```python
from build123d import *

# Parameters (mm, degrees)
SKETCH_1_W      = 20
SKETCH_1_H      = 6
SKETCH_1_W_2    = 6
SKETCH_1_H_2    = 20
EXTRUDE_1_DEPTH = 6


with BuildPart() as part:
    # Эскиз1 → Бобышка-Вытянуть1 (new body)
    with BuildSketch(Plane.XY):
        Polygon((0, 60), (0, 66), (12, 66), (12, 60), (62, 60), (62, 66), (112, 66), (112, 60), (200, 60), (200, 66), (250, 66), (250, 60), (338, 60), (338, 66), (388, 66), (388, 60), (438, 60), (438, 66), (450, 66), (450, 60), (450, 40), (438, 40), (438, 20), (450, 20), (450, 0), (450, -6), (0, -6), (0, 0), (0, 20), (12, 20), (12, 40), (0, 40), align=None)
        with Locations((62, 3)):
            Rectangle(SKETCH_1_W, SKETCH_1_H, mode=Mode.SUBTRACT)
        with Locations((225, 3)):
            Rectangle(SKETCH_1_W, SKETCH_1_H, mode=Mode.SUBTRACT)
        with Locations((388, 3)):
            Rectangle(SKETCH_1_W, SKETCH_1_H, mode=Mode.SUBTRACT)
        with Locations((29, 30)):
            Rectangle(SKETCH_1_W_2, SKETCH_1_H_2, mode=Mode.SUBTRACT)
        with Locations((421, 30)):
            Rectangle(SKETCH_1_W_2, SKETCH_1_H_2, mode=Mode.SUBTRACT)
    extrude(amount=EXTRUDE_1_DEPTH)


solid = part.part
```
Source: CAD feature listing. Evaluate the final solid. Frame: model axes, mm. Give positions to 0.01 mm unless a question says otherwise; leave off trailing zeros. Loops run counter-clockwise (first coordinate to the right, second up) from the corner with the lowest first, then second, coordinate; pieces in that order, holes last. Notation, with made-up numbers: (8, 0.25) - (16, 0.25) arc R23 cw to (16, 19.25) - close; hole circle Ø2 at (-14.5, 30). An arc over 180 degrees is marked (long way). Use CSV: the item, a comma, the result in double quotes.
1) Pin query (flat end, axial travel): P1, Ø3, axis at y = 25.5, z = 2, coming from the -X side; P2, Ø1, axis at y = 35, z = 4.5, coming from the +X side. Return the tip coordinate at first contact, or that it passes through.
Worked out:
P1,"stops at x = 12"
P2,"stops at x = 438"
2) Line query: line 1 (X direction, y = 37.5, z = 2.7); line 2 (X direction, y = 4, z = 0.85); line 3 (Y direction, x = 421.5, z = 1.6). Output: solid intervals per line, ascending.
Worked out:
line 1,"x = 12 to 26, 32 to 418, 424 to 438"
line 2,"x = 0 to 52, 72 to 215, 235 to 378, 398 to 450"
line 3,"y = -6 to 20, 40 to 60"
3) Cut plane C-C (x = 277.5). Output: boundary loops of the cut face in (y, z).
Worked out:
outline,"(-6, 0) - (60, 0) - (60, 6) - (-6, 6) - close"
4) Cut plane A-A (y = 35.5). Output: boundary loops of the cut face in (x, z), and give its area (3 significant figures).
Worked out:
outline,"(12, 0) - (26, 0) - (26, 6) - (12, 6) - close; (32, 0) - (418, 0) - (418, 6) - (32, 6) - close; (424, 0) - (438, 0) - (438, 6) - (424, 6) - close"
area,"2,480 mm^2"
5) Cut plane B-B (z = 0.95). Count the separate pieces of the cut face and the enclosed holes in it, and give its area (3 significant figures).
Worked out:
separate pieces,"1"
enclosed holes,"5"
area,"29,700 mm^2"
